```python
from build123d import *

# Parameters (mm, degrees)
BOSS_EXTRUDE1_DEPTH = 50.8
BOSS_EXTRUDE3_START = 50.8
SKETCH4_R           = 22.225
BOSS_EXTRUDE3_DEPTH = 50.8
SKETCH8_W           = 6.35
SKETCH8_H           = 36.78487194
BOSS_EXTRUDE5_DEPTH = 26.649040147
CIRPATTERN2_COUNT   = 2
CIRPATTERN2_ANGLE   = 180
SKETCH9_R           = 3.3655
CUT_EXTRUDE1_DEPTH  = 90.858670283
CUT_EXTRUDE2_REACH  = 109.65
SKETCH10_R          = 1.190625


with BuildPart() as part:
    # Sketch1 → Boss-Extrude1 (new body)
    with BuildSketch(Plane.XY):
        Polygon((-50.8, 14.559871939), (-23.859231637, 41.500640303), (23.859231637, 41.500640303), (50.8, 14.559871939), (48.55493597, 12.314807909), (22.544103576, 38.325640303), (-22.544103576, 38.325640303), (-48.55493597, 12.314807909), align=None)
    extrude(amount=BOSS_EXTRUDE1_DEPTH)

    # Sketch4 → Boss-Extrude3 (add)
    with BuildSketch(Plane.XZ.offset(-38.325640303).offset(BOSS_EXTRUDE3_START)):
        with Locations((0, 25.4)):
            Circle(SKETCH4_R)
    extrude(amount=-BOSS_EXTRUDE3_DEPTH)

    # Sketch8 → Boss-Extrude5 (add, along a direction that is not the sketch's normal)
    with BuildSketch(Plane(origin=(-30.434871939, 30.434871939, 0), x_dir=(0, 0, -1), z_dir=(0.7071067811865515, -0.7071067811865436, 0))):
        with Locations((-25.4, -7.233204333)):
            Rectangle(SKETCH8_W, SKETCH8_H)
    boss_extrude5 = extrude(amount=BOSS_EXTRUDE5_DEPTH, dir=(1, 0, 0))

    # CirPattern2: Boss-Extrude5 ×2 about axis
    cirpattern2_axis = Axis((0, 101.18743315, 25.4), (0, -1, 0))
    for i in range(1, CIRPATTERN2_COUNT):
        add(boss_extrude5.rotate(cirpattern2_axis, i * CIRPATTERN2_ANGLE / (CIRPATTERN2_COUNT - 1)))

    # Sketch9 → Cut-Extrude1 (cut, through all)
    with BuildSketch(Plane(origin=(0, 41.500640303, 0), x_dir=(1, 0, 0), z_dir=(0, 1, 0))):
        with Locations(Location((0, -25.4, 0), (0, 0, 180))):
            Circle(SKETCH9_R)
    extrude(amount=-CUT_EXTRUDE1_DEPTH, mode=Mode.SUBTRACT)

    # Sketch10 → Cut-Extrude2 (cut, up to next)
    with BuildSketch(Plane(origin=(-32.67993597, 32.67993597, 0), x_dir=(0, 0, 1), z_dir=(-0.7071067811865517, 0.7071067811865434, 0)), mode=Mode.PRIVATE) as cut_extrude2_sk1:
        with Locations(Location((15.875, -6.575640303, 0), (0, 0, 270))):
            Circle(SKETCH10_R)
    cut_extrude2_tool1 = extrude(cut_extrude2_sk1.sketch, amount=-CUT_EXTRUDE2_REACH, mode=Mode.PRIVATE) & part.part
    # Sketch10 → Cut-Extrude2 (cut, up to next)
    with BuildSketch(Plane(origin=(-32.67993597, 32.67993597, 0), x_dir=(0, 0, 1), z_dir=(-0.7071067811865517, 0.7071067811865434, 0)), mode=Mode.PRIVATE) as cut_extrude2_sk2:
        with Locations(Location((34.925, -6.575640303, 0), (0, 0, 270))):
            Circle(SKETCH10_R)
    cut_extrude2_tool2 = extrude(cut_extrude2_sk2.sketch, amount=-CUT_EXTRUDE2_REACH, mode=Mode.PRIVATE) & part.part
    cut_extrude2_1 = cut_extrude2_tool1.solids().sort_by_distance((-37.329616, 28.030256, 15.875))[0]
    add(cut_extrude2_1, mode=Mode.SUBTRACT)
    cut_extrude2_2 = cut_extrude2_tool2.solids().sort_by_distance((-37.329616, 28.030256, 34.925))[0]
    add(cut_extrude2_2, mode=Mode.SUBTRACT)
    cut_extrude2 = cut_extrude2_1 + cut_extrude2_2  # Cut-Extrude2 as one shape, for the pattern or mirror that repeats it

    # Mirror2: Cut-Extrude2 across plane
    add(cut_extrude2.mirror(Plane(origin=(0, 0, 0), x_dir=(0, 0, 1), z_dir=(1, 0, 0))), mode=Mode.SUBTRACT)


solid = part.part
```
Verification items for the finished model (mm, model axes). A direction names the side the tool comes from. Give positions to 0.01 mm unless a question says otherwise; leave off trailing zeros. Order: outer loops, then holes, each group sorted by start corner. A loop starts at its lowest first (then second) coordinate and runs counter-clockwise, first axis right, second up. Notation, with made-up numbers: (82.5, -15.75) -> (101.5, -15.75) arc R15 cw to (101.5, 11.25) -> close; hole circle Ø11 at (24, 31). An arc over 180 degrees is marked (long way). One line per item, written item: value.
(1) Sectioned sample at A-A on x = 0. Record the cut outline in (y, z) (1 decimal).
Final values:
outline: (-12.5, 3.2) -> (38.3, 3.2) -> (38.3, 0) -> (41.5, 0) -> (41.5, 22) -> (-12.5, 22) -> close; (-12.5, 28.8) -> (41.5, 28.8) -> (41.5, 50.8) -> (38.3, 50.8) -> (38.3, 47.6) -> (-12.5, 47.6) -> close
(2) Draft check along X on faces 1 (the face through (49.69, 13.45, 25.04)), 2 (the face through (31, 20, 22.225)), 3 (the face through (5, 41.501, 25)), 4 (the face through (-35.37, 25.5, 10.96)). Enter one of: pulls with the +X half, pulls with the -X half, needs draft (parallel to the pull), parting line crosses it, or undercut.
Final values:
face 1: pulls with the +X half
face 2: undercut
face 3: needs draft
face 4: undercut
(3) Scan lines: line 1 along Z through (x, y) = (0, 22) (1 decimal); line 2 along Z through (x, y) = (30.5, 28) (3 decimals); line 3 along X through (y, z) = (19, 25). Record each from-to range of solid material in increasing order. Write a range as [from, to].
Final values:
line 1: [3.2, 22], [28.8, 47.6]
line 2: [22.225, 28.575]
line 3: [-46.36, -3.34], [3.34, 46.36]
(4) Sectioned sample at D-D on x = -11. Record the cut outline in (y, z).
Final values:
outline: (-12.47, 6.09) -> (38.33, 6.09) -> (38.33, 0) -> (41.5, 0) -> (41.5, 50.8) -> (38.33, 50.8) -> (38.33, 44.71) -> (-12.47, 44.71) -> close
(5) Tool access check on faces 5 (the face through (20.53, 12.57, 16.89)), 6 (the face through (0, 38.326, 1)), 7 (the face through (31, 20, 28.575)), 8 (the face through (-35, 12.315, 25)). Record the directions out of +Z, -Z, +X, -X, +Y, -Y that give a thin tool (end or side, any length) a straight path to the whole face; none if there is none.
Final values:
face 5: -Y
face 6: -Z, -Y
face 7: +Z, -Y
face 8: +Z, -Z, -X, -Y
(6) Gauge pin test, flat ends, axial feed: pin 1 (12 mm diameter, centred on x = 25.5, z = 9.5, fed in from +Y); pin 2 (1 mm diameter, centred on x = -25.5, z = 18.5, fed in from -Y); pin 3 (1 mm diameter, centred on y = 22, z = 22, fed in from +X); pin 4 (3 mm diameter, centred on x = -27, y = 25.5, fed in from -Z) (3 decimals). Record the tip position at first contact, or that the pin passes through.
Final values:
pin 1: y = 41.5
pin 2: y = 34.87
pin 3: x = 43.86
pin 4: z = 22.225
(7) Sectioned sample at B-B on z = 25.4. Record the cut outline in (x, y) (1 decimal), then the cut area to 3 significant figures.
Final values:
outline: (-50.8, 14.6) -> (-48.6, 12.3) -> (-22.2, 12.3) -> (-22.2, -12.5) -> (-3.4, -12.5) -> (-3.4, 41.5) -> (-23.9, 41.5) -> close; (3.4, -12.5) -> (22.2, -12.5) -> (22.2, 12.3) -> (48.6, 12.3) -> (50.8, 14.6) -> (23.9, 41.5) -> (3.4, 41.5) -> close
area: 2,970 mm^2
